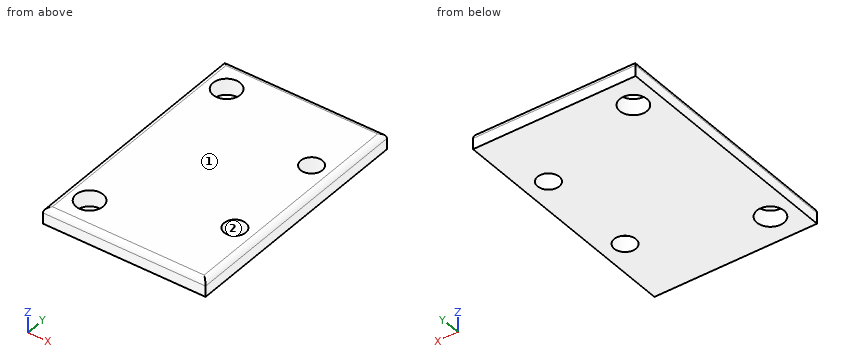
```python
from build123d import *

# Parameters (mm, degrees)
SKETCH_R   = 2
SKETCH_R_2 = 2.5
PAD_DEPTH  = 3
FILLET_R   = 1


with BuildPart() as part:
    # Sketch → Pad (new body)
    with BuildSketch(Plane.XY):
        Polygon((3.298189, -21.861723), (33.298189, -21.861723), (33.298189, -8.861723), (33.298189, 10.138277), (33.298189, 23.138277), (3.298189, 23.138277), (3.298189, 17.638277), (3.298189, -16.361723), align=None)
        with Locations((29.048189, 10.138277)):
            Circle(SKETCH_R, mode=Mode.SUBTRACT)
        with Locations((29.048189, -8.861723)):
            Circle(SKETCH_R, mode=Mode.SUBTRACT)
        with Locations((7.798189, -16.361723)):
            Circle(SKETCH_R_2, mode=Mode.SUBTRACT)
        with Locations((7.798189, 17.638277)):
            Circle(SKETCH_R_2, mode=Mode.SUBTRACT)
    extrude(amount=PAD_DEPTH)

    # Fillet
    fillet_edges = [part.edges().sort_by_distance(p)[0] for p in [
        (18.298189, 23.138277, 3),
        (33.298189, 0.638277, 3),
        (33.298189, 16.638277, 3),
        (33.298189, -15.361723, 3),
        (18.298189, -21.861723, 3),
        (3.298189, 0.638277, 3),
        (3.298189, 20.388277, 3),
        (3.298189, -19.111723, 3),
    ]]
    fillet(fillet_edges, radius=FILLET_R)


solid = part.part
```
Can you work these out from the model? Positions are in its coordinate system, mm. Face numbers are marked on the shaded views. Round coordinates to 2 decimals unless told otherwise and drop trailing zeros. Loops run counter-clockwise (first coordinate to the right, second up) from the corner with the lowest first, then second, coordinate; pieces in that order, holes last. Notation, with made-up numbers: (47.25, 75.5) -> (74.25, 75.5) arc R27 cw to (74.25, 95.5) -> close; hole circle Ø6 at (-17.75, 7). An arc over 180 degrees is marked (long way). One line per item, written item: value. Start each with the question number.
1. If I drill on probe 1 along Y at (x, z) = (9.75, 1.05); probe 2 along Y at (x, z) = (30.5, 1.3); probe 3 along Y at (x, z) = (23.75, 2.45), over which ranges is the centre line in solid material (lowest first)?
2. If we section it at C-C, the plane z = 0.9: Write out the boundary of the cut face in (x, y).
3. If we mould it in two halves opening along X, with no side actions, what happens to the marked faces 1 and 2? For each: pulls with the +X half, pulls with the -X half, needs draft (parallel to the pull), parting line crosses it, or undercut.
4. If we section it at B-B, the plane x = 8: Write out the boundary of the cut face in (y, z), then the cut area to 3 significant figures.
5. For pin 1 (2.5 mm diameter, centred on x = 29.05, y = 10.14, fed in from -Z), with a flat end and sliding along its axis, tell me the tip position at first contact or that it passes through.
6. If we section it at A-A, the plane y = -7.5: Write out the boundary of the cut face in (x, z), then the cut area to 3 significant figures.
Calculated:
1. probe 1: y = -21.86 to -17.92, -14.8 to 16.08, 19.2 to 23.14
1. probe 2: y = -21.86 to -10.24, -7.49 to 8.76, 11.51 to 23.14
1. probe 3: y = -21.75 to 23.03
2. outline: (3.3, -21.86) -> (33.3, -21.86) -> (33.3, 23.14) -> (3.3, 23.14) -> close; hole circle Ø5 at (7.8, -16.36); hole circle Ø5 at (7.8, 17.64); hole circle Ø4 at (29.05, -8.86); hole circle Ø4 at (29.05, 10.14)
3. face 1: needs draft
3. face 2: undercut
4. outline: (-21.86, 0) -> (-18.85, 0) -> (-18.85, 3) -> (-20.86, 3) arc R1 ccw to (-21.86, 2) -> close; (-13.87, 0) -> (15.15, 0) -> (15.15, 3) -> (-13.87, 3) -> close; (20.13, 0) -> (23.14, 0) -> (23.14, 2) arc R1 ccw to (22.14, 3) -> (20.13, 3) -> close
4. area: 105 mm²
5. pin 1: passes through
6. outline: (3.3, 0) -> (27.58, 0) -> (27.58, 3) -> (4.3, 3) arc R1 ccw to (3.3, 2) -> close; (30.51, 0) -> (33.3, 0) -> (33.3, 2) arc R1 ccw to (32.3, 3) -> (30.51, 3) -> close
6. area: 80.8 mm²
